Source: CAD feature listing. Evaluate the final solid. Frame: model axes, mm. A direction names the side the tool comes from. Coordinates: 2 decimals unless noted, no trailing zeros. Order: outer loops, then holes, each group sorted by start corner. A loop starts at its lowest first (then second) coordinate and runs counter-clockwise, first axis right, second up. Notation, with made-up numbers: (38, 13.5) -> (77, 13.5) arc R18 cw to (77, 30.5) -> close; hole circle Ø5 at (14.5, 14). An arc over 180 degrees is marked (long way). Put each result on its own line as item: value.
from build123d import *

# Parameters (mm, degrees)
SKETCH1_W           = 230
SKETCH1_H           = 100
SKETCH1_R           = 2.285
BOSS_EXTRUDE1_DEPTH = 8


with BuildPart() as part:
    # Sketch1 → Boss-Extrude1 (new body)
    with BuildSketch(Plane.XY):
        Rectangle(SKETCH1_W, SKETCH1_H)
        with Locations((-97, 10)):
            Circle(SKETCH1_R, mode=Mode.SUBTRACT)
        with Locations((-97, -35)):
            Circle(SKETCH1_R, mode=Mode.SUBTRACT)
        with Locations((-75, -40)):
            Circle(SKETCH1_R, mode=Mode.SUBTRACT)
        with Locations(Location((75, -40, 0), (0, 0, 180))):
            Circle(SKETCH1_R, mode=Mode.SUBTRACT)
        with Locations(Location((97, -35, 0), (0, 0, 180))):
            Circle(SKETCH1_R, mode=Mode.SUBTRACT)
        with Locations(Location((97, 10, 0), (0, 0, 180))):
            Circle(SKETCH1_R, mode=Mode.SUBTRACT)
        with Locations((75, 40)):
            Circle(SKETCH1_R, mode=Mode.SUBTRACT)
        with Locations(Location((-75, 40, 0), (0, 0, 180))):
            Circle(SKETCH1_R, mode=Mode.SUBTRACT)
        with BuildLine():
            Line((-84.52993562, 1.412877308), (-1.993630557, 37.298227335))
            ThreePointArc((-1.993630557, 37.298227335), (4.585350281, 34.706507611), (1.993630557, 28.127526773))
            Line((1.993630557, 28.127526773), (-80.542674506, -7.757823255))
            ThreePointArc((-80.542674506, -7.757823255), (-87.121655344, -5.166103531), (-84.52993562, 1.412877308))
        make_face(mode=Mode.SUBTRACT)
        with BuildLine():
            Line((-43.261783088, -13.357324732), (39.274521974, 22.528025295))
            ThreePointArc((39.274521974, 22.528025295), (45.853502813, 19.936305571), (43.261783088, 13.357324732))
            Line((43.261783088, 13.357324732), (-39.274521974, -22.528025295))
            ThreePointArc((-39.274521974, -22.528025295), (-45.853502813, -19.936305571), (-43.261783088, -13.357324732))
        make_face(mode=Mode.SUBTRACT)
        with BuildLine():
            Line((-1.993630557, -28.127526773), (80.542674506, 7.757823255))
            ThreePointArc((80.542674506, 7.757823255), (87.121655344, 5.166103531), (84.52993562, -1.412877308))
            Line((84.52993562, -1.412877308), (1.993630557, -37.298227335))
            ThreePointArc((1.993630557, -37.298227335), (-4.585350281, -34.706507611), (-1.993630557, -28.127526773))
        make_face(mode=Mode.SUBTRACT)
    extrude(amount=BOSS_EXTRUDE1_DEPTH)


solid = part.part
1. Cut plane D-D on y = -25.5. Output: boundary loops of the cut face in (x, z), plus the area to 3 significant figures.
Numbers:
outline: (-115, 0) -> (4.05, 0) -> (4.05, 8) -> (-115, 8) -> close; (29.13, 0) -> (115, 0) -> (115, 8) -> (29.13, 8) -> close
area: 1,640 mm2
2. First-contact query: pin 1 (3.5 mm diameter, centred on x = 97, y = -35, fed in from +Z). Flat tip, straight axial feed; report the tip coordinate or a pass-through.
Numbers:
pin 1: passes through
3. Ray query, line 1 along Y through (x, z) = (-97, 6) (3 decimals); line 2 along X through (y, z) = (17.5, 5); line 3 along X through (y, z) = (-33.5, 6.5). Return the intervals inside material, ascending.
Numbers:
line 1: y = -50 to -37.285, -32.715 to 7.715, 12.285 to 50
line 2: x = -115 to -47.53, -22.45 to 27.71, 46.25 to 115
line 3: x = -115 to -98.72, -95.28 to -4.94, 10.73 to 95.28, 98.72 to 115
4. Cut plane B-B on z = 6.5. Count the separate pieces of the cut face and the enclosed holes in it, plus the area to 3 significant figures.
Numbers:
separate pieces: 1
enclosed holes: 11
area: 19,900 mm2
5. Cut plane C-C on x = 55. Output: boundary loops of the cut face in (y, z), plus the area to 3 significant figures.
Numbers:
outline: (-50, 0) -> (-14.25, 0) -> (-14.25, 8) -> (-50, 8) -> close; (-3.35, 0) -> (50, 0) -> (50, 8) -> (-3.35, 8) -> close
area: 713 mm2
6. Set-up query: faces 1 (the flat face through (-2, -50, 4)), 2 (the flat face through (-2.571, 4.334, 3.944)). Return all of +Z, -Z, +X, -X, +Y, -Y with unobstructed straight access to the full face (end or side cutting, diameter ignored); none if empty.
Numbers:
face 1: +Z, -Z, +X, -X, -Y
face 2: +Z, -Z
7. Cut plane A-A on y = 40. Output: boundary loops of the cut face in (x, z) (3 decimals), plus the area to 3 significant figures.
Numbers:
outline: (-115, 0) -> (-77.285, 0) -> (-77.285, 8) -> (-115, 8) -> close; (-72.715, 0) -> (72.715, 0) -> (72.715, 8) -> (-72.715, 8) -> close; (77.285, 0) -> (115, 0) -> (115, 8) -> (77.285, 8) -> close
area: 1,770 mm2
